Check sheet for the modelled part. Datum: model origin and axes. Units: mm. Face numbers are marked on the shaded views. Round coordinates to 2 decimals unless told otherwise and drop trailing zeros. Write each loop counter-clockwise with the first axis right and the second up, starting at its lowest first coordinate (ties: lowest second). Pieces come first, ordered by that corner, then holes.
Item 1: Section check C-C, the plane z = -1.8. Record the cut outline in (x, y).
Item 2: Release check for a two-part mould opening along X. For the marked faces 1, 2, 3 and 4 record: pulls with the +X half, pulls with the -X half, needs draft (parallel to the pull), parting line crosses it, or undercut.
Item 3: Section check B-B, the plane y = 2.75. State how many separate pieces and enclosed holes the cut face has, plus the area to 3 significant figures.
Item 4: Depth check by flat-ended pin: pin 1 (0.7 mm diameter, centred on x = -11.5, y = 5, fed in from -Z); pin 2 (0.7 mm diameter, centred on y = -2, z = -4, fed in from +X); pin 3 (0.7 mm diameter, centred on x = -4, y = -2, fed in from +Z). Enter the tip coordinate at first touch or a pass-through.
Item 5: Section check A-A, the plane x = -10. Record the cut outline in (y, z), plus the area to 3 significant figures.
Item 6: Material ranges on line 1 along X through (y, z) = (4, -1.3); line 2 along Z through (x, y) = (-11.5, -1.5); line 3 along Y through (x, z) = (-1.5, -1.9), recorded low to high.
Autodesk Inventor part; units mm, degrees
ref_plane "YZ Plane" through (0, 0, 0) normal (1, 0, 0) x (0, 1, 0)
ref_plane "XZ Plane" through (0, 0, 0) normal (0, 1, 0) x (-1, 0, 0)
ref_plane "XY Plane" through (0, 0, 0) normal (0, 0, 1) x (1, 0, 0)
sketch "Sketch1" plane through (0, 0, 0) normal (0, 1, 0) x (-1, 0, 0)
  line L0 (0, 0) -> (12.7, 0)
  line L1 (12.7, 0) -> (12.7, -5.08)
  line L2 (12.7, -5.08) -> (0, -5.08)
  line L3 (0, -5.08) -> (0, 0)
  dimension "d0" = 12.7
  dimension "d1" = 5.08
extrude "Extrusion1" add sketch "Sketch1" along normal blind 2.4
chamfer "Chamfer1" distance 0.2 angle 45 4 edges at (-12.7, 1.2, -5.08) (-12.7, 1.2, 0) (0, 1.2, 0) (0, 1.2, -5.08)
sketch "Sketch2" plane through (0, 2.4, 0) normal (0, 1, 0) x (1, 0, 0)
  line L0 (-11.13, 0.97) -> (-11.73, 0.97)
  line L1 (-11.73, 0.97) -> (-11.73, 1.57)
  line L2 (-11.73, 1.57) -> (-11.13, 1.57)
  line L3 (-11.13, 1.57) -> (-11.13, 0.97)
  line L4 (-11.13, 0.97) -> (-11.73, 1.57) construction
  line L5 (-11.73, 0.97) -> (-11.13, 1.57) construction
  line L6 (-11.13, 3.51) -> (-11.73, 3.51)
  line L7 (-11.73, 3.51) -> (-11.73, 4.11)
  line L8 (-11.73, 4.11) -> (-11.13, 4.11)
  line L9 (-11.13, 4.11) -> (-11.13, 3.51)
  line L10 (-11.13, 3.51) -> (-11.73, 4.11) construction
  line L11 (-11.73, 3.51) -> (-11.13, 4.11) construction
  line L12 (-8.59, 0.97) -> (-9.19, 0.97)
  line L13 (-9.19, 0.97) -> (-9.19, 1.57)
  line L14 (-9.19, 1.57) -> (-8.59, 1.57)
  line L15 (-8.59, 1.57) -> (-8.59, 0.97)
  line L16 (-8.59, 0.97) -> (-9.19, 1.57) construction
  line L17 (-9.19, 0.97) -> (-8.59, 1.57) construction
  line L18 (-8.59, 3.51) -> (-9.19, 3.51)
  line L19 (-9.19, 3.51) -> (-9.19, 4.11)
  line L20 (-9.19, 4.11) -> (-8.59, 4.11)
  line L21 (-8.59, 4.11) -> (-8.59, 3.51)
  line L22 (-8.59, 3.51) -> (-9.19, 4.11) construction
  line L23 (-9.19, 3.51) -> (-8.59, 4.11) construction
  line L24 (-6.05, 0.97) -> (-6.65, 0.97)
  line L25 (-6.65, 0.97) -> (-6.65, 1.57)
  line L26 (-6.65, 1.57) -> (-6.05, 1.57)
  line L27 (-6.05, 1.57) -> (-6.05, 0.97)
  line L28 (-6.05, 0.97) -> (-6.65, 1.57) construction
  line L29 (-6.65, 0.97) -> (-6.05, 1.57) construction
  line L30 (-6.05, 3.51) -> (-6.65, 3.51)
  line L31 (-6.65, 3.51) -> (-6.65, 4.11)
  line L32 (-6.65, 4.11) -> (-6.05, 4.11)
  line L33 (-6.05, 4.11) -> (-6.05, 3.51)
  line L34 (-6.05, 3.51) -> (-6.65, 4.11) construction
  line L35 (-6.65, 3.51) -> (-6.05, 4.11) construction
  line L36 (-3.51, 0.97) -> (-4.11, 0.97)
  line L37 (-4.11, 0.97) -> (-4.11, 1.57)
  line L38 (-4.11, 1.57) -> (-3.51, 1.57)
  line L39 (-3.51, 1.57) -> (-3.51, 0.97)
  line L40 (-3.51, 0.97) -> (-4.11, 1.57) construction
  line L41 (-4.11, 0.97) -> (-3.51, 1.57) construction
  line L42 (-3.51, 3.51) -> (-4.11, 3.51)
  line L43 (-4.11, 3.51) -> (-4.11, 4.11)
  line L44 (-4.11, 4.11) -> (-3.51, 4.11)
  line L45 (-3.51, 4.11) -> (-3.51, 3.51)
  line L46 (-3.51, 3.51) -> (-4.11, 4.11) construction
  line L47 (-4.11, 3.51) -> (-3.51, 4.11) construction
  line L48 (-0.97, 0.97) -> (-1.57, 0.97)
  line L49 (-1.57, 0.97) -> (-1.57, 1.57)
  line L50 (-1.57, 1.57) -> (-0.97, 1.57)
  line L51 (-0.97, 1.57) -> (-0.97, 0.97)
  line L52 (-0.97, 0.97) -> (-1.57, 1.57) construction
  line L53 (-1.57, 0.97) -> (-0.97, 1.57) construction
  line L54 (-0.97, 3.51) -> (-1.57, 3.51)
  line L55 (-1.57, 3.51) -> (-1.57, 4.11)
  line L56 (-1.57, 4.11) -> (-0.97, 4.11)
  line L57 (-0.97, 4.11) -> (-0.97, 3.51)
  line L58 (-0.97, 3.51) -> (-1.57, 4.11) construction
  line L59 (-1.57, 3.51) -> (-0.97, 4.11) construction
  line L60 (-12.7, 4.88) -> (-12.7, 0.2)
  line L61 (-12.5, 0) -> (-0.2, 0)
  point P0 (0, 0)
  point P1 (-11.43, 1.27)
  point P2 (-11.43, 3.81)
  point P3 (-8.89, 1.27)
  point P4 (-8.89, 3.81)
  point P5 (-6.35, 1.27)
  point P6 (-6.35, 3.81)
  point P7 (-3.81, 1.27)
  point P8 (-3.81, 3.81)
  point P9 (-1.27, 1.27)
  point P10 (-1.27, 3.81)
  dimension "d7" = 0.6
  dimension "d8" = 0.6
  dimension "d11" = 2.54
  dimension "d14" = 2.54
  dimension "d17" = 1.27
  dimension "d18" = 1.27
extrude "Extrusion2" add sketch "Sketch2" along normal blind 6.1 and the other way blind 5.2
properties part number "2x5_P2.54mm_male_header"
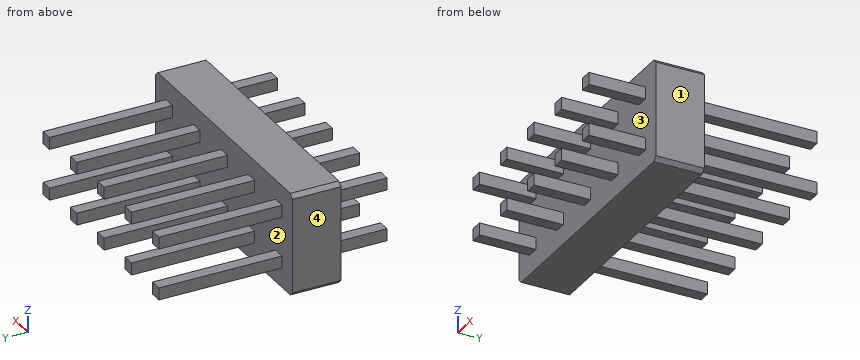
Values found:
1. outline: (-12.7, 0) - (0, 0) - (0, 2.4) - (-12.7, 2.4) - close
2. face 1: pulls with the +X half
2. face 2: undercut
2. face 3: undercut
2. face 4: pulls with the -X half
3. separate pieces: 10
3. enclosed holes: 0
3. area: 3.60 mm2
4. pin 1: stops at z = -4.11
4. pin 2: stops at x = -0.97
4. pin 3: stops at z = -0.97
5. outline: (0, -5.08) - (2.4, -5.08) - (2.4, 0) - (0, 0) - close
5. area: 12.2 mm2
6. line 1: x = -11.73 to -11.13, -9.19 to -8.59, -6.65 to -6.05, -4.11 to -3.51, -1.57 to -0.97
6. line 2: z = -4.11 to -3.51, -1.57 to -0.97
6. line 3: y = 0 to 2.4
